Here's how the part is built. I have some questions about the finished solid (model axes, mm). Face numbers are marked on the shaded views. A direction names the side the tool comes from. Give positions to 0.01 mm unless a question says otherwise; leave off trailing zeros. Loops run counter-clockwise (first coordinate to the right, second up) from the corner with the lowest first, then second, coordinate; pieces in that order, holes last. Notation, with made-up numbers: (-15, 37) - (29, 37) arc R23 cw to (29, 73) - close; hole circle Ø9 at (63, 73.25). An arc over 180 degrees is marked (long way). Return JSON: item names as keys, results as strings. Group by question number.
(1) If we section it at B-B (x = -50): Please give me the cut outline in (y, z).
(2) I need wall thicknesses on probe 1 along X at (y, z) = (6.25, -42.5); probe 2 along X at (y, z) = (8, -30); probe 3 along X at (y, z) = (3.5, -30). Which ranges of each line are inside material? Lowest first, please. Write a range as [from, to].
(3) If we mould it in two halves opening along X, with no side actions, what happens to the marked faces 3, 4, 5 and 6? For each: released by +X, released by -X, zero draft, split by the parting line, or undercut.
(4) For P1, Ø1, axis at x = -50, y = 6, coming from the -Z side; P2, Ø1.5, axis at x = -108, y = 4, coming from the -Z side; P3, Ø1, axis at x = -62, y = 7.5, coming from the -Z side, each with a flat end and sliding along its axis, tell me the tip position at first contact or that it passes through.
(5) If we section it at A-A (z = -68): Please give me the cut outline in (x, y).
(6) On a 3-axis mill with a long thin cutter (end or side, diameter ignored), from which of +Z, -Z, +X, -X, +Y, -Y can I reach the whole of each face in a straight line? I mean the marked faces 1 and 2. Say none if no direction works.
(7) If we section it at D-D (z = -105): Please give me the cut outline in (x, y), then the cut area to 3 significant figures.
(8) If we section it at C-C (x = -105): State how many separate pieces and enclosed holes the cut face has, then the cut area to 3 significant figures.
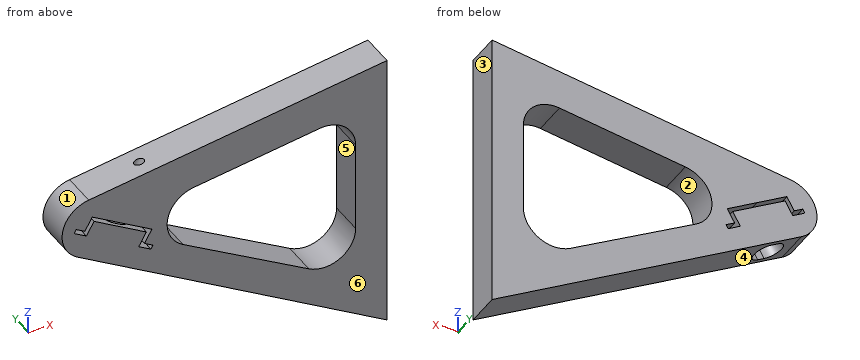
Autodesk Inventor part; units mm, degrees
ref_plane "YZ Plane" through (0, 0, 0) normal (1, 0, 0) x (0, 1, 0)
ref_plane "XZ Plane" through (0, 0, 0) normal (0, 1, 0) x (-1, 0, 0)
ref_plane "XY Plane" through (0, 0, 0) normal (0, 0, 1) x (1, 0, 0)
sketch "Sketch1" plane through (0, 0, 0) normal (0, 1, 0) x (-1, 0, 0)
  line L0 (0, 0) -> (0, -114.3)
  line L1 (0, -114.3) -> (125.3564, -41.9254)
  line L2 (0, -114.3) -> (144.7491, -114.3) construction
  line L3 (120.9141, -18.371) -> (0, 0)
  arc A0 (125.3564, -41.9254) -> (120.9141, -18.371) centre (119.0064, -30.9269) ccw
  line L4 (12.7, -32.7621) -> (12.7, -69.4305)
  line L5 (0, -114.3) -> (0, -98.425)
  line L6 (31.6623, -80.4792) -> (82.681, -51.5623)
  line L7 (78.3264, -27.9577) -> (27.3077, -20.2062)
  arc A1 (82.681, -51.5623) -> (78.3264, -27.9577) centre (76.4188, -40.5136) ccw
  arc A2 (12.7, -69.4305) -> (31.6623, -80.4792) centre (25.4, -69.4305) ccw
  arc A3 (27.3077, -20.2062) -> (12.7, -32.7621) centre (25.4, -32.7621) ccw
  line L8 (126.7827, -31.0259) -> (121.8464, -33.8759)
  line L9 (121.8464, -33.8759) -> (118.7464, -28.5065)
  line L10 (126.7827, -31.0259) -> (125.9327, -29.5536)
  line L11 (125.9327, -29.5536) -> (122.4686, -31.5536)
  line L12 (122.4686, -31.5536) -> (119.4686, -26.3575)
  line L13 (118.7464, -28.5065) -> (108.1376, -34.6315)
  line L14 (119.4686, -26.3575) -> (107.3876, -33.3325)
  line L15 (95.6924, -48.9759) -> (100.6288, -46.1259)
  line L16 (100.6288, -46.1259) -> (97.5288, -40.7565)
  line L17 (95.6924, -48.9759) -> (94.8424, -47.5036)
  line L18 (94.8424, -47.5036) -> (98.3065, -45.5036)
  line L19 (98.3065, -45.5036) -> (95.3065, -40.3075)
  line L20 (97.5288, -40.7565) -> (108.1376, -34.6315)
  line L21 (95.3065, -40.3075) -> (107.3876, -33.3325)
  point P0 (156.7289, -23.8125)
  dimension "d0" = 114.3
  dimension "d2" = 30
  dimension "d3" = 12.7
  dimension "d5" = 15.875
  dimension "d8" = 12.7
  dimension "d9" = 12.7
  dimension "d34" = 5.7
  dimension "d36" = 6.2
  dimension "d37" = 1.7
  dimension "d38" = 4
  dimension "d39" = 6
  dimension "d41" = 12.25
  dimension "d42" = 13.95
  dimension "d45" = 1.7
  dimension "d46" = 12.25
  dimension "d47" = 13.95
  dimension "d48" = 1.7
  dimension "d49" = 6.2
  dimension "d50" = 5.7
  dimension "d59" = 24.5
extrude "Extrusion2" add sketch "Sketch1" along normal blind 14
sketch "Sketch3" plane through (-97.5288, 0, -40.7565) normal (0.5, 0, 0.866) x (0.866, 0, -0.5)
  line L0 (-13.75, 7) -> (-10.75, 7) construction
  line L1 (-13.75, 2) -> (-10.75, 2)
  line L2 (-10.75, 12) -> (-13.75, 12)
  arc A0 (-13.75, 12) -> (-13.75, 2) centre (-13.75, 7) ccw
  arc A1 (-10.75, 2) -> (-10.75, 12) centre (-10.75, 7) ccw
  line L3 (0, 0) -> (-24.5, 0)
  line L4 (-24.5, 0) -> (-24.5, 14)
  point P0 (64.0841, 0)
  point P1 (-12.25, 7)
  dimension "d55" = 10
  dimension "d56" = 7
  dimension "d57" = 3
  dimension "d58" = 12.25
extrude "Extrusion3" cut sketch "Sketch3" against normal up to next
sketch "Sketch4" plane through (-125.3564, 0, -41.9254) normal (-0.5, 0, -0.866) x (-0.866, 0, 0.5)
  arc A0 (-9.765, 2) -> (-9.765, 12) centre (-9.765, 7) ccw
  arc A1 (-12.765, 12) -> (-12.765, 2) centre (-12.765, 7) ccw
  line L0 (-9.765, 12) -> (-12.765, 12)
  line L1 (-9.765, 2) -> (-12.765, 2)
  line L2 (-9.765, 12) -> (-12.765, 2)
  line L3 (-9.765, 2) -> (-12.765, 12)
  circle A2 centre (-11.265, 7) radius 1.65
  point P0 (-87.5991, 0)
  dimension "d62" = 3.3
extrude "Extrusion4" cut sketch "Sketch4" against normal up to next contours A2 L2 L3 | L3 L2 A2 | L2 L3 A2 | A2 L3 L2
properties part number "Din_Rail_0.45mm_Clearance"
Values:
{
 "1": {"outline": "(0, -85.43) - (14, -85.43) - (14, -70.09) - (0, -70.09) - close; (0, -23.65) - (14, -23.65) - (14, -7.6) - (0, -7.6) - close"},
 "2": {"probe 1": "[-124.36, -120.12], [-105.24, -98.54], [-96.57, -88.96], [-12.7, 0]", "probe 2": "[-131.67, -126.19], [-125.16, -121.57], [-119.61, -116.16], [-113.16, -106.98], [-103.95, -83.54], [-13, 0]", "probe 3": "[-131.67, -126.19], [-125.16, -121.57], [-119.61, -116.16], [-113.16, -83.54], [-13, 0]"},
 "3": {"face 3": "released by +X", "face 4": "released by -X", "face 5": "undercut", "face 6": "zero draft"},
 "4": {"P1": "z = -85.72", "P2": "z = -52.38", "P3": "z = -78.79"},
 "5": {"outline": "(-80.19, 0) - (-53.68, 0) - (-53.68, 14) - (-80.19, 14) - close; (-12.7, 0) - (0, 0) - (0, 14) - (-12.7, 14) - close"},
 "6": {"face 1": "-X, +Y, -Y", "face 2": "+Y, -Y"},
 "7": {"outline": "(-16.11, 0) - (0, 0) - (0, 14) - (-16.11, 14) - close", "area": "226 mm2"},
 "8": {"separate pieces": "2", "enclosed holes": "1", "area": "449 mm2"}
}
